from build123d import *

# Parameters (mm, degrees)
SKETCH_W       = 31.75
SKETCH_H       = 31.75
SKETCH_W_2     = 26.2128
SKETCH_H_2     = 26.2128
PAD_DEPTH      = 254
PAD_DEPTH_BACK = 254
POCKET_DEPTH   = 31.75


with BuildPart() as part:
    # Sketch → Pad (new body, two sides)
    with BuildSketch(Plane.YZ) as pad_sk:
        Rectangle(SKETCH_W, SKETCH_H)
        Rectangle(SKETCH_W_2, SKETCH_H_2, mode=Mode.SUBTRACT)
    extrude(amount=PAD_DEPTH)
    extrude(pad_sk.sketch, amount=-PAD_DEPTH_BACK)

    # Sketch002 → Pocket (cut)
    with BuildSketch(Plane(origin=(0, 0, 15.875), x_dir=(0, -1, 0), z_dir=(0, 0, 1))):
        Polygon((15.875, -254), (-15.875, -254), (-15.875, -231.115916), align=None)
    pocket = extrude(amount=-POCKET_DEPTH, mode=Mode.SUBTRACT)

    # Mirrored: Pocket across Sketch002 H_Axis
    add(pocket.mirror(Plane(origin=(0, 0, 15.875), x_dir=(0, 0, 1), z_dir=(1, 0, 0))), mode=Mode.SUBTRACT)


solid = part.part
Design review of the part built by this model. Coordinates are the model's own, in mm. A direction names the side the tool comes from. Give positions to 0.01 mm unless a question says otherwise; leave off trailing zeros. Loops run counter-clockwise (first coordinate to the right, second up) from the corner with the lowest first, then second, coordinate; pieces in that order, holes last. Notation, with made-up numbers: M 2,27.25 L 23,27.25 A32 cw 23,62.25 Z; hole C 5.5,13 d2. An arc over 180 degrees is marked long. One line per question, with ' | ' between items. Start each with the question number.
1. To check wall thickness, follow L1, parallel to Y at x = -55.5, z = -13 (3 decimals); L2, parallel to Y at x = -231.5, z = 3.5 (3 decimals). State the ranges of each line that lie inside material, in increasing order.
2. For faces 1 (the face through (-242.4, 0.22, -13.89)), 2 (the face through (4, -13.106, 0)), list the 3-axis set-ups (+Z, -Z, +X, -X, +Y, -Y) from which the entire face can be reached by the end or side of a thin tool; tool diameter is ignored.
3. Add section A-A (x = 65.5). Write out the cut boundary in (y, z) (3 decimals).
4. Add section C-C (z = 5). Write out the cut boundary in (x, y) (1 decimal), plus the area to 3 significant figures.
5. The part is to be moulded in two halves that separate along Y. For faces 3 (the face through (4, 0, -13.106)), 4 (the face through (4, 0, 15.875)), 5 (the face through (4, -15.875, 0)), 6 (the face through (3, 15.875, 0)), say which applies: released by +Y, released by -Y, zero draft, split by the parting line, or undercut.
6. Insertion check: P1, Ø8, axis at y = 4.5, z = -12, coming from the +X side; P2, Ø10, axis at y = -3.5, z = -11, coming from the +X side; P3, Ø1, axis at y = -11.5, z = 3.5, coming from the -X side. Each pin has a flat end and moves straight along its axis. Give the tip position at first contact, or say it passes through.
7. Add section B-B (y = 1). Write out the cut boundary in (x, z) (3 decimals).
Worked out:
1) L1: y = -15.875 to -13.106, 13.106 to 15.875 | L2: y = -15.875 to -13.106, 13.106 to 15.342
2) face 1: +Z, -Z, -X, +Y | face 2: +X, -X
3) outline: M -15.875,-15.875 L 15.875,-15.875 L 15.875,15.875 L -15.875,15.875 Z; hole M -13.106,-13.106 L 13.106,-13.106 L 13.106,13.106 L -13.106,13.106 Z
4) outline: M -254,-15.9 L 254,-15.9 L 252,-13.1 L -252,-13.1 Z; M -233.1,13.1 L 233.1,13.1 L 231.1,15.9 L -231.1,15.9 Z | area: 2,690 mm²
5) face 3: undercut | face 4: zero draft | face 5: released by -Y | face 6: released by +Y
6) P1: stops at x = 242.09 | P2: stops at x = 248.35 | P3: passes through
7) outline: M -241.837,-15.875 L 241.837,-15.875 L 241.837,-13.106 L -241.837,-13.106 Z; M -241.837,13.106 L 241.837,13.106 L 241.837,15.875 L -241.837,15.875 Z
